Design review of the part built by this model. Coordinates are the model's own, in mm. Face numbers are marked on the shaded views. Round coordinates to 2 decimals unless told otherwise and drop trailing zeros. Write each loop counter-clockwise with the first axis right and the second up, starting at its lowest first coordinate (ties: lowest second). Pieces come first, ordered by that corner, then holes.
Autodesk Inventor part; units mm, degrees
ref_plane "YZ Plane" through (0, 0, 0) normal (1, 0, 0) x (0, 1, 0)
ref_plane "XZ Plane" through (0, 0, 0) normal (0, 1, 0) x (-1, 0, 0)
ref_plane "XY Plane" through (0, 0, 0) normal (0, 0, 1) x (1, 0, 0)
sketch "Esboço1" plane through (0, 0, 0) normal (0, 0, 1) x (1, 0, 0)
  line L0 (0, 0) -> (110, 0)
  line L1 (110, 0) -> (110, 15)
  line L2 (110, 15) -> (0, 15)
  line L3 (0, 15) -> (0, 0)
  dimension "d0" = 110
  dimension "d1" = 15
extrude "Extrusão1" add sketch "Esboço1" along normal blind 15
chamfer "Chanfro1" distance 10 distance2 32 1 edges at (110, 15, 7.5) measured on face at (110, 5, 5)
sketch "Esboço2" plane through (0, 0, 0) normal (0, -1, 0) x (1, 0, 0)
  line L0 (0, 15) -> (110, 15)
  line L1 (0, 0) -> (0, 15)
  point P0 (13, 7.5)
  dimension "d7" = 7.5
  dimension "d8" = 13
hole "Furo1" at (13, 0, 7.5) direction (0, 1, 0) diameter 8 depth 10.4 tip angle 118
sketch "Esboço3" plane through (0, 0, 0) normal (0, -1, 0) x (1, 0, 0)
  point P0 (0, 0)
sketch "Esboço4" plane through (0, 0, 0) normal (0, -1, 0) x (1, 0, 0)
  circle A0 centre (13, 7.5) radius 4
  point P0 (0, 0)
  point P1 (66, 7.5)
  dimension "d17" = 53
hole "Furo2" at (66, 0, 7.5) direction (0, 1, 0) diameter 11 end through all
properties part number "Garra1"
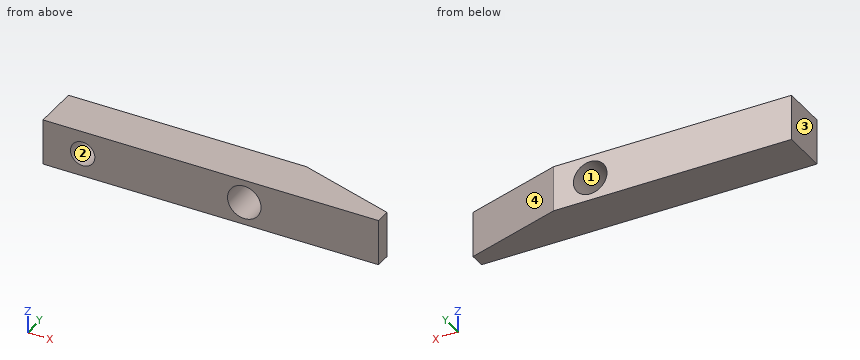
1) For line 1 along Z through (x, y) = (66, 3.5); line 2 along X through (y, z) = (3.75, 7.5); line 3 along Z through (x, y) = (13, 6), list the stretches that pass through material, from the lowest coordinate up.
2) Add section A-A on x = 66. State the section outline as (y, z) points, and give its area (3 significant figures).
3) The part is to be moulded in two halves that separate along X. For the marked faces 1, 2, 3 and 4, say which applies: pulls with the +X half, pulls with the -X half, needs draft (parallel to the pull), parting line crosses it, or undercut.
4) Add section B-B on y = 11.5. State the section outline as (x, z) points.
Computed:
1. line 1: z = 0 to 2, 13 to 15
1. line 2: x = 0 to 9, 17 to 60.5, 71.5 to 110
1. line 3: z = 0 to 3.5, 11.5 to 15
2. outline: (0, 0) - (15, 0) - (15, 2) - (0, 2) - close; (0, 13) - (15, 13) - (15, 15) - (0, 15) - close
2. area: 60.0 mm2
3. face 1: undercut
3. face 2: undercut
3. face 3: pulls with the -X half
3. face 4: pulls with the +X half
4. outline: (0, 0) - (89.2, 0) - (89.2, 15) - (0, 15) - close; hole circle Ø4.34 at (13, 7.5); hole circle Ø11 at (66, 7.5)
